Here's the drawing with two shaded views (mm, measured from the low corner). I have some questions. A direction names the side the tool comes from. Round coordinates to 2 decimals unless told otherwise and drop trailing zeros. Loops run counter-clockwise (first coordinate to the right, second up) from the corner with the lowest first, then second, coordinate; pieces in that order, holes last.
(1) If I drill on line 1 along X through (y, z) = (106.5, 51); line 2 along Y through (x, z) = (39.5, 37); line 3 along Z through (x, y) = (47.5, 5.5), over which ranges is the centre line in solid material (lowest first)?
(2) I want a section at A-A on y = 19.5. Write out the boundary of the cut face in (x, z).
(3) Which directions (+Z, -Z, +X, -X, +Y, -Y) give clear straight access to the entire face, cutting with the end or side of a thin tool? Please do the marked faces 1 and 2.
(4) Will this pin go through, and if not, where does the flat tip stop? pin 1 Ø10 at (x, y) = (11, 96.5) entering from +Z.
(5) I want a section at B-B on x = 63.5. Write out the boundary of the cut face in (y, z), plus the area to 3 significant figures.
(6) I want a section at C-C on z = 30. Write out the boundary of the cut face in (x, y).
(7) Thinking about a two-plate mould opening in Y: for the marked faces 3, 4, 5 and 6, which applies, released by +Y, released by -Y, zero draft, split by the parting line, or undercut?
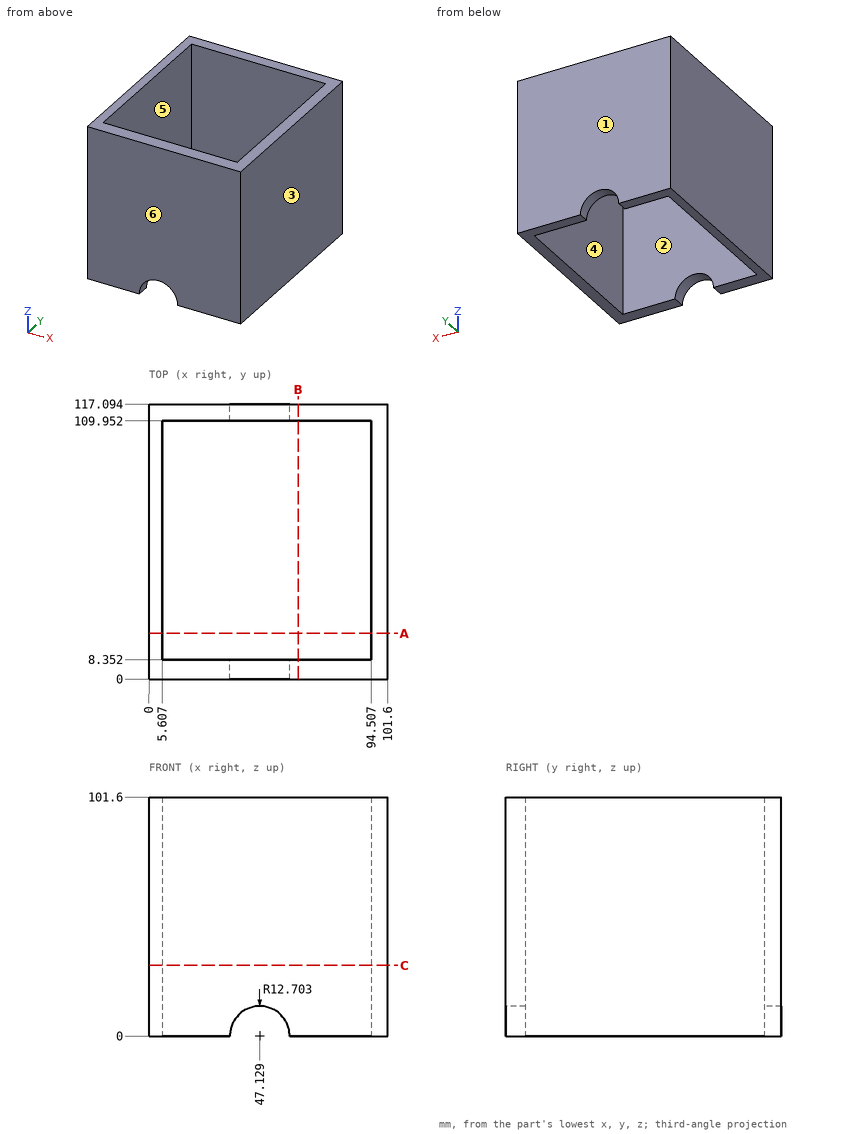
Filled sheet:
1. line 1: x = 0 to 5.61, 94.51 to 101.6
1. line 2: y = 0 to 8.35, 109.95 to 117.09
1. line 3: z = 12.7 to 101.6
2. outline: (0, 0) - (5.61, 0) - (5.61, 101.6) - (0, 101.6) - close; (94.51, 0) - (101.6, 0) - (101.6, 101.6) - (94.51, 101.6) - close
3. face 1: +Z, -Z, +X, -X, +Y
3. face 2: +Z, -Z
4. pin 1: passes through
5. outline: (0, 0) - (8.35, 0) - (8.35, 101.6) - (0, 101.6) - close; (109.95, 0) - (117.09, 0) - (117.09, 101.6) - (109.95, 101.6) - close
5. area: 1,570 mm2
6. outline: (0, 0) - (101.6, 0) - (101.6, 117.09) - (0, 117.09) - close; hole (5.61, 8.35) - (94.51, 8.35) - (94.51, 109.95) - (5.61, 109.95) - close
7. face 3: zero draft
7. face 4: undercut
7. face 5: undercut
7. face 6: released by -Y
